For this review, use the dimensioned drawing (mm, ordinates from the lowest corner) and the shaded views. Coordinates: 2 decimals unless noted, no trailing zeros. Loops run counter-clockwise (first coordinate to the right, second up) from the corner with the lowest first, then second, coordinate; pieces in that order, holes last. Notation, with made-up numbers: (50, 9) - (72, 9) arc R6 cw to (72, 13) - close; hole circle Ø10 at (-21, -38). An arc over 180 degrees is marked (long way). Use a Markdown table: item, result. Add a question column.
1) Add section B-B, the plane z = 25. Give the boundary of the cut face in (x, y).
2) Add section D-D, the plane x = 24. Give the boundary of the cut face in (y, z).
3) To check wall thickness, follow L1, parallel to X at y = 48.5, z = 15.5; L2, parallel to X at y = 72.5, z = 5; L3, parallel to Y at x = 64.5, z = 12. State the ranges of each line that lie inside material, in increasing order. Write a range as [from, to].
4) The part is to be moulded in two halves that separate along X. For the marked faces 1, 2 and 3, say which applies: pulls with the +X half, pulls with the -X half, needs draft (parallel to the pull), parting line crosses it, or undercut.
5) Add section C-C, the plane x = 67. Give the boundary of the cut face in (y, z) (3 decimals), and give its area (3 significant figures).
6) Add section A-A, the plane y = 50.8. Give the boundary of the cut face in (x, z) (3 decimals).
7) Clearance check with flat-ended pins moving along their axes: pin 1 (25 mm diameter, centred on x = 22.225, y = 22.225, fed in from +Z); pin 2 (5 mm diameter, centred on x = 85, y = 13.5, fed in from -Z); pin 3 (15 mm diameter, centred on y = 44, z = 22.5, fed in from +X); pin 4 (1.9 mm diameter, centred on x = 66, z = 14, fed in from +Y). State where each tip first meets the part, or that it passes through.
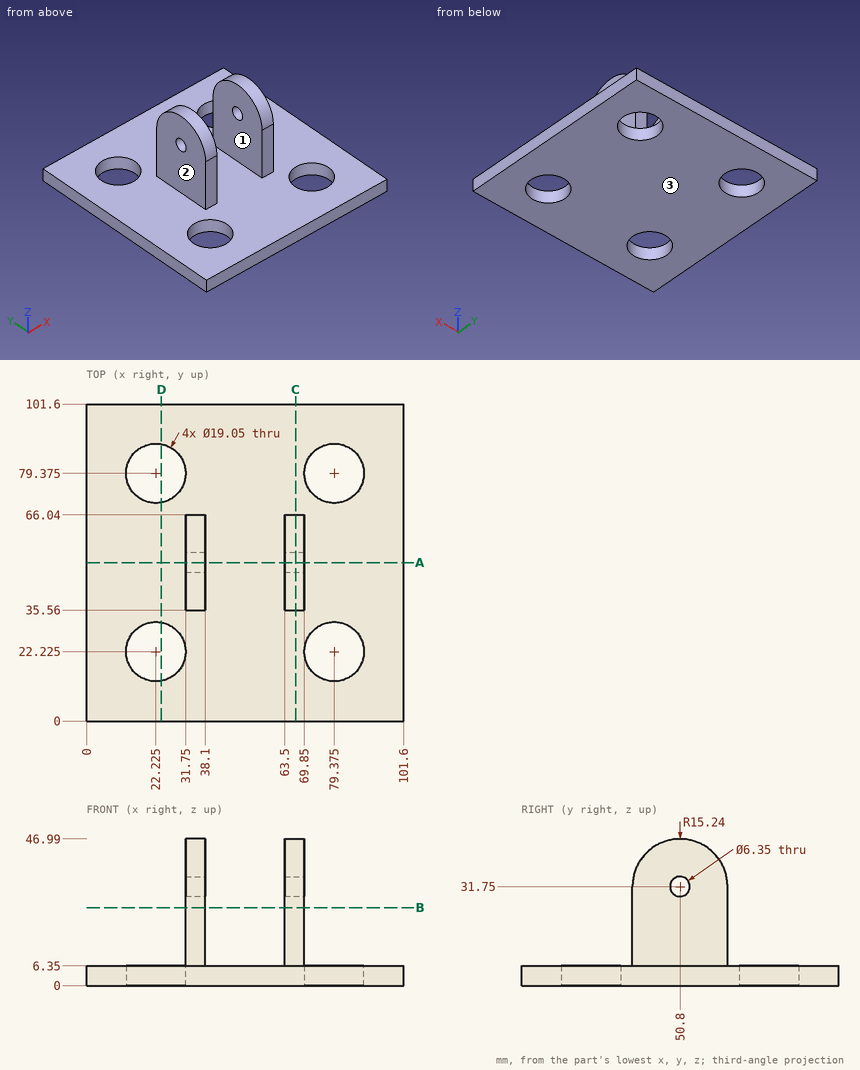
From the geometry:
| question | item | result |
|---|---|---|
| 1 | outline | (31.75, 35.56) - (38.1, 35.56) - (38.1, 66.04) - (31.75, 66.04) - close; (63.5, 35.56) - (69.85, 35.56) - (69.85, 66.04) - (63.5, 66.04) - close |
| 2 | outline | (0, 0) - (12.87, 0) - (12.87, 6.35) - (0, 6.35) - close; (31.58, 0) - (70.02, 0) - (70.02, 6.35) - (31.58, 6.35) - close; (88.73, 0) - (101.6, 0) - (101.6, 6.35) - (88.73, 6.35) - close |
| 3 | L1 | x = [31.75, 38.1], [63.5, 69.85] |
| 3 | L2 | x = [0, 15.63], [28.82, 72.78], [85.97, 101.6] |
| 3 | L3 | y = [35.56, 66.04] |
| 4 | face 1 | undercut |
| 4 | face 2 | pulls with the -X half |
| 4 | face 3 | needs draft |
| 5 | outline | (0, 0) - (101.6, 0) - (101.6, 6.35) - (66.04, 6.35) - (66.04, 31.75) arc R15.24 ccw to (35.56, 31.75) - (35.56, 6.35) - (0, 6.35) - close; hole circle Ø6.35 at (50.8, 31.75) |
| 5 | area | 1,750 mm^2 |
| 6 | outline | (0, 0) - (101.6, 0) - (101.6, 6.35) - (69.85, 6.35) - (69.85, 28.575) - (63.5, 28.575) - (63.5, 6.35) - (38.1, 6.35) - (38.1, 28.575) - (31.75, 28.575) - (31.75, 6.35) - (0, 6.35) - close; (31.75, 34.925) - (38.1, 34.925) - (38.1, 46.99) - (31.75, 46.99) - close; (63.5, 34.925) - (69.85, 34.925) - (69.85, 46.99) - (63.5, 46.99) - close |
| 7 | pin 1 | stops at z = 6.35 |
| 7 | pin 2 | stops at z = 0 |
| 7 | pin 3 | stops at x = 69.85 |
| 7 | pin 4 | stops at y = 66.04 |
